Geometry check sheet. Reference: the model listing, model coordinates, mm. Face numbers are marked on the shaded views. A direction names the side the tool comes from. Give positions to 0.01 mm unless a question says otherwise; leave off trailing zeros. Loops run counter-clockwise (first coordinate to the right, second up) from the corner with the lowest first, then second, coordinate; pieces in that order, holes last. Notation, with made-up numbers: (-1, 53.25) -> (39, 53.25) arc R13 cw to (39, 75.25) -> close; hole circle Ø6 at (28, 59.5). An arc over 180 degrees is marked (long way). Write each question's results on one line, items separated by ' | '. Start each with the question number.
1) Set-up check for the marked faces 4 and 5: record each of +Z, -Z, +X, -X, +Y, -Y from which the full face is reachable in a straight line by a thin tool's end or side.
2) Sectioned sample at B-B on z = 384.5. Record the cut outline in (x, y), then the cut area to 3 significant figures.
3) Scan lines: line 1 (X direction, y = -209, z = 409.5); line 2 (Y direction, x = -57.5, z = 240.5). Record each from-to range of solid material in increasing order. Write a range as from..to.
4) Sectioned sample at C-C on x = -42. Record the cut outline in (y, z).
5) Sectioned sample at A-A on y = -44. Record the cut outline in (x, z).
6) Depth check by flat-ended pin: pin 1 (4 mm diameter, centred on x = -128.5, z = 191.5, fed in from -Y); pin 2 (12 mm diameter, centred on x = -125, y = -56, fed in from +Z). Enter the tip coordinate at first touch or a pass-through.
7) Draft check along X on the marked faces 1, 2 and 3. Enter one of: pulls with the +X half, pulls with the -X half, needs draft (parallel to the pull), parting line crosses it, or undercut.
```python
from build123d import *

# Parameters (mm, degrees)
F1_DEPTH = 426
F2_W     = 295
F2_H     = 360
F3_DEPTH = 4
F4_R     = 2


# Not quite as in the source:
# - a feature names something its author has since deleted; it is built from what else it names


with BuildPart() as f1:
    # F0 (on Top) → F1 (new body)
    with BuildSketch(Plane.XY):
        Polygon((-4, -360), (0, -360), (0, 0), (-295, 0), (-295, -360), (-291, -360), (-291, -4), (-4, -4), align=None)
    extrude(amount=F1_DEPTH)

    # F2 (on Top) → F3 (join)
    with BuildSketch(Plane.XY):
        with Locations((-147.5, -180)):
            Rectangle(F2_W, F2_H)
    extrude(amount=-F3_DEPTH)

    # F4
    f4_edges = [f1.edges().sort_by_distance(p)[0] for p in [
        (-295, -180, -4),
        (0, -180, -4),
    ]]
    fillet(f4_edges, radius=F4_R)


solid = f1.part
```
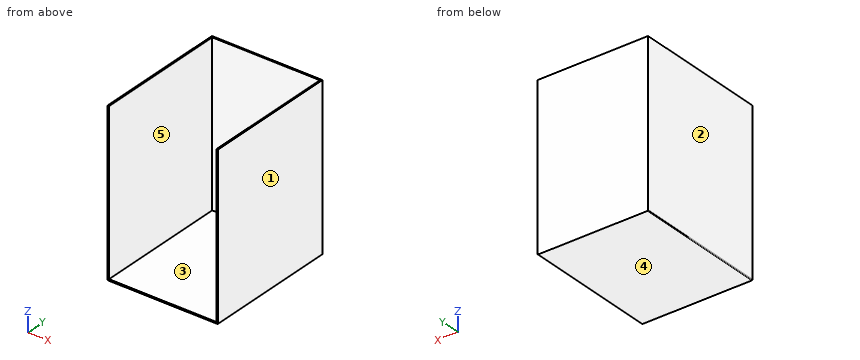
Result:
1) face 4: -Z, +X, -X, +Y, -Y | face 5: +Z, -Y
2) outline: (-295, -360) -> (-291, -360) -> (-291, -4) -> (-4, -4) -> (-4, -360) -> (0, -360) -> (0, 0) -> (-295, 0) -> close | area: 4,030 mm^2
3) line 1: -295..-291, -4..0 | line 2: -4..0
4) outline: (-360, -4) -> (0, -4) -> (0, 426) -> (-4, 426) -> (-4, 0) -> (-360, 0) -> close
5) outline: (-295, -2) arc R2 ccw to (-293, -4) -> (-2, -4) arc R2 ccw to (0, -2) -> (0, 426) -> (-4, 426) -> (-4, 0) -> (-291, 0) -> (-291, 426) -> (-295, 426) -> close
6) pin 1: y = -4 | pin 2: z = 0
7) face 1: pulls with the +X half | face 2: pulls with the -X half | face 3: undercut
